```python
from build123d import *

# Parameters (mm, degrees)
CYLINDER040_R     = 0.75
CYLINDER040_DEPTH = 10
CYLINDER037_R     = 0.75
CYLINDER037_DEPTH = 10
BOX038_W          = 5
BOX038_H          = 10
BOX038_DEPTH      = 3
BOX003_W          = 4
BOX003_H          = 19
BOX003_DEPTH      = 5
FILLET_R          = 1
FILLET001_R       = 1
FILLET002_R       = 1
FILLET003_R       = 1


with BuildPart() as cilindro040:
    # Cylinder040 → Cylinder040 (new body)
    with BuildSketch(Plane(origin=(-26, 66, 42), x_dir=(1, 0, 0), z_dir=(0, 0, 1))):
        Circle(CYLINDER040_R)
    extrude(amount=CYLINDER040_DEPTH)


with BuildPart() as cilindro037:
    # Cylinder037 → Cylinder037 (new body)
    with BuildSketch(Plane(origin=(-26, 53, 42), x_dir=(1, 0, 0), z_dir=(0, 0, 1))):
        Circle(CYLINDER037_R)
    extrude(amount=CYLINDER037_DEPTH)


with BuildPart() as cubo038:
    # Box038 → Box038 (new body)
    with BuildSketch(Plane(origin=(-28.5, 54.5, 51), x_dir=(1, 0, 0), z_dir=(0, 0, 1))):
        with Locations((2.5, 5)):
            Rectangle(BOX038_W, BOX038_H)
    extrude(amount=BOX038_DEPTH)


with BuildPart() as cut058:
    # Box003 → Box003 (new body)
    with BuildSketch(Plane(origin=(-2, 50, 45), x_dir=(1, 0, 0), z_dir=(0, 0, 1))):
        with Locations((2, 9.5)):
            Rectangle(BOX003_W, BOX003_H)
    extrude(amount=BOX003_DEPTH)

    # Fillet
    fillet_edges = [cut058.edges().sort_by_distance(p)[0] for p in [
        (2, 59.5, 50),
    ]]
    fillet(fillet_edges, radius=FILLET_R)

    # Fillet001
    fillet001_edges = [cut058.edges().sort_by_distance(p)[0] for p in [
        (-2, 59.5, 50),
    ]]
    fillet(fillet001_edges, radius=FILLET001_R)

    # Fillet002
    fillet002_edges = [cut058.edges().sort_by_distance(p)[0] for p in [
        (0, 69, 50),
    ]]
    fillet(fillet002_edges, radius=FILLET002_R)

    # Fillet003
    fillet003_edges = [cut058.edges().sort_by_distance(p)[0] for p in [
        (0, 50, 50),
    ]]
    fillet(fillet003_edges, radius=FILLET003_R)


with BuildPart() as cut058_1:
    # Fillet003 placement: moved
    add(cut058.part.moved(Location((-26, 0, 6))))

    # Cut055: cut Cubo038
    add(cubo038.part, mode=Mode.SUBTRACT)


with BuildPart() as cut058_2:
    # Cut055 placement: moved
    add(cut058_1.part.moved(Location((0, 0, -6))))

    # Cut057: cut Cilindro037
    add(cilindro037.part, mode=Mode.SUBTRACT)

    # Cut058: cut Cilindro040
    add(cilindro040.part, mode=Mode.SUBTRACT)


with BuildPart() as cut058_3:
    # Cut058 placement: moved
    add(cut058_2.part.moved(Location((0, 0.5, 0))))


solid = cut058_3.part
```
Here's how the part is built. I have some questions about the finished solid (model axes, mm). A direction names the side the tool comes from. Give positions to 0.01 mm unless a question says otherwise; leave off trailing zeros. Write each loop counter-clockwise with the first axis right and the second up, starting at its lowest first coordinate (ties: lowest second). Pieces come first, ordered by that corner, then holes. Notation, with made-up numbers: (-37.5, -28) -> (-6.5, -28) arc R14 cw to (-6.5, -15) -> close; hole circle Ø8 at (-39.5, -24.5). An arc over 180 degrees is marked (long way). Use one line per item in the form item = value.
1) Suppose I cut it at C-C (z = 48.2). Please give me the cut outline in (x, y).
Verdict:
outline = (-28, 51.5) arc R1 ccw to (-27, 50.5) -> (-25, 50.5) arc R1 ccw to (-24, 51.5) -> (-24, 68.5) arc R1 ccw to (-25, 69.5) -> (-27, 69.5) arc R1 ccw to (-28, 68.5) -> close; hole circle Ø1.5 at (-26, 53.5); hole circle Ø1.5 at (-26, 66.5)
2) We'd pull the mould along Y, two halves only. Please class faces 1 (the face through (-27.715, 50.801, 47.028)), 2 (the face through (-26, 52, 45)), 3 (the face through (-26, 60, 48)): +Y half, -Y half, draft (parallel to the pull), parting line (faces both ways), or undercut.
Verdict:
face_1 = -Y half
face_2 = draft
face_3 = undercut
3) Suppose I cut it at B-B (x = -26). Please give me the cut outline in (y, z), and give its area (3 significant figures).
Verdict:
outline = (50.5, 45) -> (52.75, 45) -> (52.75, 50) -> (51.5, 50) arc R1 ccw to (50.5, 49) -> close; (54.25, 45) -> (55, 45) -> (55, 48) -> (65, 48) -> (65, 45) -> (65.75, 45) -> (65.75, 50) -> (54.25, 50) -> close; (67.25, 45) -> (69.5, 45) -> (69.5, 49) arc R1 ccw to (68.5, 50) -> (67.25, 50) -> close
area = 49.6 mm2
4) On a 3-axis mill with a long thin cutter (end or side, diameter ignored), from which of +Z, -Z, +X, -X, +Y, -Y can I reach the whole of each face in a straight line? I mean faces 4 (the face through (-25.986, 50.801, 49.715)), 5 (the face through (-26, 65, 46)). Say none if no direction works.
Verdict:
face_4 = +Z, +X, -X, -Y
face_5 = -Z, +X, -X
5) Suppose I cut it at A-A (z = 45.75). Please give me the cut outline in (x, y), and give its area (3 significant figures).
Verdict:
outline = (-28, 51.5) arc R1 ccw to (-27, 50.5) -> (-25, 50.5) arc R1 ccw to (-24, 51.5) -> (-24, 55) -> (-28, 55) -> close; (-28, 65) -> (-24, 65) -> (-24, 68.5) arc R1 ccw to (-25, 69.5) -> (-27, 69.5) arc R1 ccw to (-28, 68.5) -> close; hole circle Ø1.5 at (-26, 53.5); hole circle Ø1.5 at (-26, 66.5)
area = 31.6 mm2
6) Suppose I cut it at D-D (y = 53.5). Please give me the cut outline in (x, z), and give its area (3 significant figures).
Verdict:
outline = (-28, 45) -> (-26.75, 45) -> (-26.75, 50) -> (-27, 50) arc R1 ccw to (-28, 49) -> close; (-25.25, 45) -> (-24, 45) -> (-24, 49) arc R1 ccw to (-25, 50) -> (-25.25, 50) -> close
area = 12.1 mm2
7) If I drill on L1, parallel to Y at x = -26, z = 48.45; L2, parallel to Y at x = -26, z = 47.25; L3, parallel to Y at x = -26.45, z = 45.4, over which ranges is the centre line in solid material (lowest first)? Write a range as [from, to].
Verdict:
L1 = [50.5, 52.75], [54.25, 65.75], [67.25, 69.5]
L2 = [50.5, 52.75], [54.25, 55], [65, 65.75], [67.25, 69.5]
L3 = [50.5, 52.9], [54.1, 55], [65, 65.9], [67.1, 69.5]
